```python
from build123d import *

# Parameters (mm, degrees)
SKETCH_1_W             = 25
SKETCH_1_H             = 41
EXTRUDE_415_DEPTH      = 2
SKETCH_5_W             = 25
SKETCH_5_H             = 2
EXTRUDE_624_DEPTH      = 18.5
SKETCH_7_W             = 4
SKETCH_7_H             = 37
SKETCH_7_W_2           = 2
EXTRUDE_1265_DEPTH     = 18.5
SKETCH_8_R             = 18.5
CUT_EXTRUDE_1405_DEPTH = 2
SKETCH_9_R             = 16.5
CUT_EXTRUDE_1536_DEPTH = 23
SKETCH_10_W            = 5
SKETCH_10_H            = 37
CUT_EXTRUDE_1762_DEPTH = 2


with BuildPart() as part:
    # 草图1 → Extrude 415 (new body)
    with BuildSketch(Plane(origin=(0, 0, 0), x_dir=(1, 0, 0), z_dir=(0, 1, 0))):
        with Locations((12.5, 20.5)):
            Rectangle(SKETCH_1_W, SKETCH_1_H)
    extrude(amount=EXTRUDE_415_DEPTH)

    # 草图5 → Extrude 624 (add)
    with BuildSketch(Plane(origin=(0, 2, 0), x_dir=(1, 0, 0), z_dir=(0, 1, 0))):
        with Locations((12.5, 40)):
            Rectangle(SKETCH_5_W, SKETCH_5_H)
        with Locations((12.5, 1)):
            Rectangle(SKETCH_5_W, SKETCH_5_H)
    extrude(amount=EXTRUDE_624_DEPTH)

    # 草图7 → Extrude 1265 (add)
    with BuildSketch(Plane(origin=(0, 2, 0), x_dir=(1, 0, 0), z_dir=(0, 1, 0))):
        with Locations((2, 20.5)):
            Rectangle(SKETCH_7_W, SKETCH_7_H)
        with Locations((10, 20.5)):
            Rectangle(SKETCH_7_W_2, SKETCH_7_H)
        with Locations((17, 20.5)):
            Rectangle(SKETCH_7_W_2, SKETCH_7_H)
        with Locations((24, 20.5)):
            Rectangle(SKETCH_7_W_2, SKETCH_7_H)
    extrude(amount=EXTRUDE_1265_DEPTH)

    # 草图8 → Cut-Extrude 1405 (cut)
    with BuildSketch(Plane.ZY):
        with Locations((-20.5, 20.5)):
            Circle(SKETCH_8_R)
    extrude(amount=-CUT_EXTRUDE_1405_DEPTH, mode=Mode.SUBTRACT)

    # 草图9 → Cut-Extrude 1536 (cut)
    with BuildSketch(Plane(origin=(25, 0, 0), x_dir=(0, 0, -1), z_dir=(1, 0, 0))):
        with Locations((20.5, 20.5)):
            Circle(SKETCH_9_R)
    extrude(amount=-CUT_EXTRUDE_1536_DEPTH, mode=Mode.SUBTRACT)

    # 草图10 → Cut-Extrude 1762 (cut)
    with BuildSketch(Plane(origin=(0, 2, 0), x_dir=(1, 0, 0), z_dir=(0, 1, 0))):
        with Locations((6.5, 20.5)):
            Rectangle(SKETCH_10_W, SKETCH_10_H)
        with Locations((13.5, 20.5)):
            Rectangle(SKETCH_10_W, SKETCH_10_H)
        with Locations((20.5, 20.5)):
            Rectangle(SKETCH_10_W, SKETCH_10_H)
    extrude(amount=-CUT_EXTRUDE_1762_DEPTH, mode=Mode.SUBTRACT)


solid = part.part
```
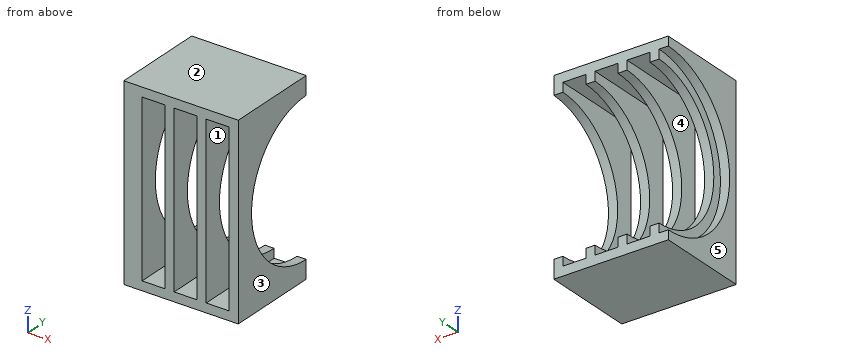
Geometry check sheet. Reference: the model listing, model coordinates, mm. Face numbers are marked on the shaded views. A direction names the side the tool comes from. Give positions to 0.01 mm unless a question says otherwise; leave off trailing zeros. Loops run counter-clockwise (first coordinate to the right, second up) from the corner with the lowest first, then second, coordinate; pieces in that order, holes last. Notation, with made-up numbers: M 26,18.5 L 53,18.5 A33 cw 53,53.5 Z; hole C 34.25,1 d10. An arc over 180 degrees is marked long. Write item = value, one per line. Start each with the question number.
1. Section check D-D, the plane x = 3.5. Enter the section's corners in (y, z), plus the area to 3 significant figures.
2. Tool access check on the marked faces 4 and 5. Record the directions out of +Z, -Z, +X, -X, +Y, -Y that give a thin tool (end or side, any length) a straight path to the whole face; none if there is none.
3. Go/stop test with flat-tipped pins: P1, Ø3, axis at x = 18, z = -7.5, coming from the +Y side; P2, Ø10.5, axis at y = 8, z = -18, coming from the -X side; P3, Ø12, axis at y = 13, z = -19, coming from the -X side. Record where each tip stops, or that it passes through.
4. Section check A-A, the plane z = -20.5. Enter the section's corners in (x, y).
5. Section check C-C, the plane z = -8. Enter the section's corners in (x, y).
6. Draft check along Z on the marked faces 1, 2 and 3. Enter one of: +Z half, -Z half, draft (parallel to the pull), parting line (faces both ways), or undercut.
7. Section check B-B, the plane x = 7.5. Enter the section's corners in (y, z).
8. Thickness scan on probe 1 along X at (y, z) = (1.75, -7.5); probe 2 along X at (y, z) = (3.5, -20.5); probe 3 along Z at (x, y) = (15, 15.25). Record the ranges inside material, lowest first.
Values follow:
q1.outline = M 0,-41 L 20.5,-41 L 20.5,-37 A16.5 cw 20.5,-4 L 20.5,0 L 0,0 Z
q1.area = 413 mm^2
q2.face_4 = +Y, -Y
q2.face_5 = +Z, -Z, -X, +Y, -Y
q3.P1 = 12.63
q3.P2 = 2
q3.P3 = through
q4.outline = M 0,0 L 4,0 L 4,4 L 2,4 L 2,2 L 0,2 Z; M 9,0 L 11,0 L 11,4 L 9,4 Z; M 16,0 L 18,0 L 18,4 L 16,4 Z; M 23,0 L 25,0 L 25,4 L 23,4 Z
q5.outline = M 0,0 L 4,0 L 4,9.73 L 2,9.73 L 2,6.86 L 0,6.86 Z; M 9,0 L 11,0 L 11,9.73 L 9,9.73 Z; M 16,0 L 18,0 L 18,9.73 L 16,9.73 Z; M 23,0 L 25,0 L 25,9.73 L 23,9.73 Z
q6.face_1 = undercut
q6.face_2 = +Z half
q6.face_3 = draft
q7.outline = M 0,-41 L 20.5,-41 L 20.5,-39 L 0,-39 Z; M 0,-2 L 20.5,-2 L 20.5,0 L 0,0 Z
q8.probe_1 = 0 to 4, 9 to 11, 16 to 18, 23 to 25
q8.probe_2 = 2 to 4, 9 to 11, 16 to 18, 23 to 25
q8.probe_3 = -41 to -39, -2 to 0
